Geometry check sheet. Reference: drawing and pictorial views, mm from the part's lowest x, y, z. Give positions to 0.01 mm unless a question says otherwise; leave off trailing zeros. Loops run counter-clockwise (first coordinate to the right, second up) from the corner with the lowest first, then second, coordinate; pieces in that order, holes last. Notation, with made-up numbers: (46.5, -36.5) -> (101.5, -36.5) arc R27 ccw to (101.5, -0.5) -> close; hole circle Ø6 at (57, -7). An arc over 180 degrees is marked (long way). One line per item, written item: value. Start each with the question number.
(1) Gauge pin test, flat ends, axial feed: pin 1 Ø1.5 at (y, z) = (20, 58.5) entering from +X; pin 2 Ø6 at (x, z) = (93, 34) entering from +Y; pin 3 Ø2 at (x, y) = (87.5, 8.5) entering from +Z; pin 4 Ø1.5 at (x, z) = (64, 42.5) entering from -Y. Record the tip position at first contact, or that the pin passes through.
(2) Sectioned sample at C-C, the plane x = 93. Record the cut outline in (y, z).
(3) Sectioned sample at B-B, the plane x = 74.5. Record the cut outline in (y, z) (1 decimal).
(4) Sectioned sample at A-A, the plane z = 68. Record the cut outline in (x, y) (1 decimal), then the cut area to 3 significant figures.
(5) Scan lines: line 1 along Z through (x, y) = (73, 6); line 2 along Y through (x, z) = (40, 107); line 3 along Z through (x, y) = (82.5, 13) (1 decimal). Record each from-to range of solid material in increasing order. Write a range as from..to.
(6) Draft check along X on the marked faces 1, 2, 3 and 4. Enter one of: pulls with the +X half, pulls with the -X half, needs draft (parallel to the pull), parting line crosses it, or undercut.
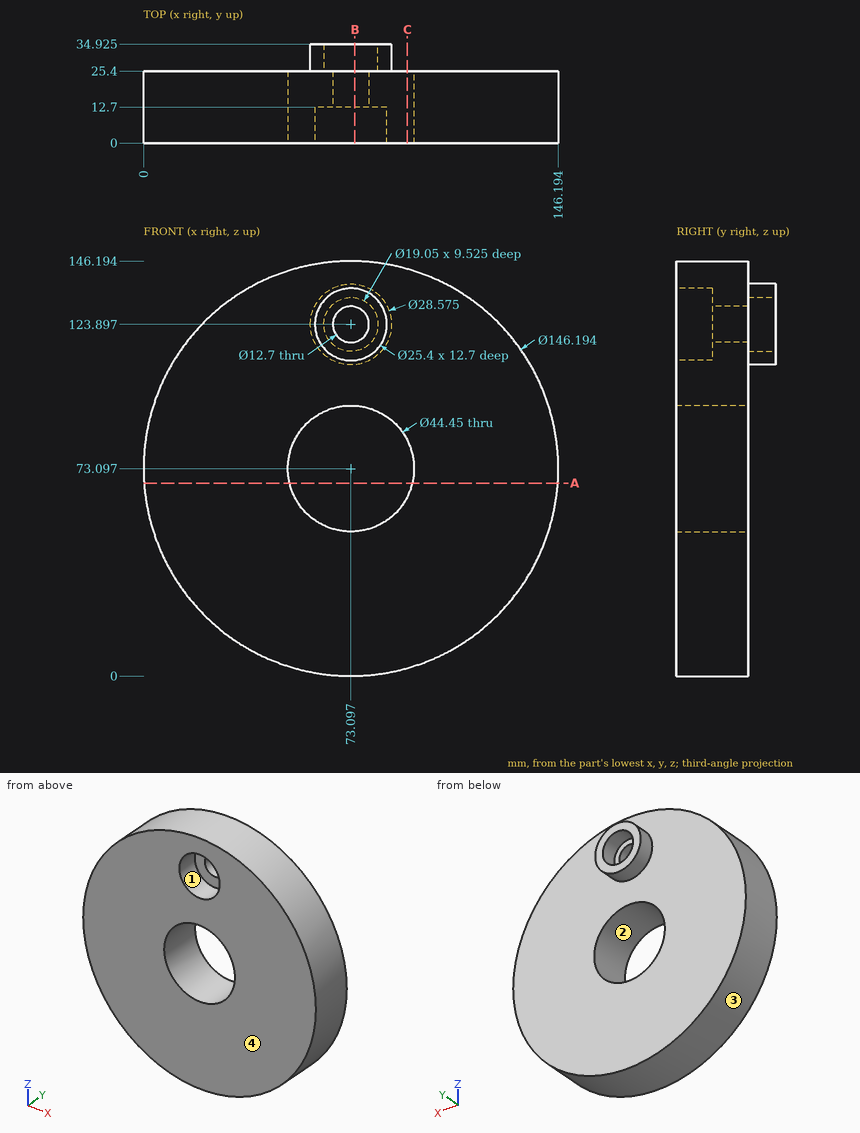
Calculated:
1. pin 1: stops at x = 144.87
1. pin 2: stops at y = 25.4
1. pin 3: stops at z = 144.95
1. pin 4: stops at y = 0
2. outline: (0, 2.76) -> (25.4, 2.76) -> (25.4, 63.21) -> (0, 63.21) -> close; (0, 82.99) -> (25.4, 82.99) -> (25.4, 143.43) -> (0, 143.43) -> close
3. outline: (0, 0) -> (25.4, 0) -> (25.4, 50.9) -> (0, 50.9) -> close; (0, 95.3) -> (25.4, 95.3) -> (25.4, 109.7) -> (34.9, 109.7) -> (34.9, 114.5) -> (25.4, 114.5) -> (25.4, 117.7) -> (12.7, 117.7) -> (12.7, 111.3) -> (0, 111.3) -> close; (0, 136.5) -> (12.7, 136.5) -> (12.7, 130.1) -> (25.4, 130.1) -> (25.4, 133.3) -> (34.9, 133.3) -> (34.9, 138.1) -> (25.4, 138.1) -> (25.4, 146.2) -> (0, 146.2) -> close
4. outline: (0.2, 0) -> (51.5, 0) -> (51.5, 25.4) -> (0.2, 25.4) -> close; (94.7, 0) -> (146, 0) -> (146, 25.4) -> (94.7, 25.4) -> close
4. area: 2,610 mm2
5. line 1: z = 0..50.87, 95.32..111.2, 136.6..146.19
5. line 2: y = 0..25.4
5. line 3: z = 0.6..53, 93.2..145.6
6. face 1: undercut
6. face 2: undercut
6. face 3: parting line crosses it
6. face 4: needs draft
